```python
from build123d import *

# Parameters (mm, degrees)
SKETCH1_R           = 6.5
SKETCH1_R_2         = 1.5
BOSS_EXTRUDE1_DEPTH = 1.5875
FILLET1_R           = 5


with BuildPart() as part:
    # Sketch1 → Boss-Extrude1 (new body)
    with BuildSketch(Plane.XY):
        Polygon((0, 0), (0, 55), (30, 55), (30, -8.038475773), (-1.519237886, -62.631397208), (-27.5, -47.631397208), align=None)
        with Locations((15, -4.019237886)):
            Circle(SKETCH1_R, mode=Mode.SUBTRACT)
        with Locations((5, 50)):
            Circle(SKETCH1_R_2, mode=Mode.SUBTRACT)
        with Locations((5, 30)):
            Circle(SKETCH1_R_2, mode=Mode.SUBTRACT)
        with Locations((5, 10)):
            Circle(SKETCH1_R_2, mode=Mode.SUBTRACT)
        with Locations(Location((25, 10, 0), (0, 0, 180))):
            Circle(SKETCH1_R_2, mode=Mode.SUBTRACT)
        with Locations(Location((25, 30, 0), (0, 0, 180))):
            Circle(SKETCH1_R_2, mode=Mode.SUBTRACT)
        with Locations(Location((25, 50, 0), (0, 0, 180))):
            Circle(SKETCH1_R_2, mode=Mode.SUBTRACT)
        with Locations((-20.669872981, -45.801270189)):
            Circle(SKETCH1_R_2, mode=Mode.SUBTRACT)
        with Locations((-10.669872981, -28.480762114)):
            Circle(SKETCH1_R_2, mode=Mode.SUBTRACT)
        with Locations((-0.669872981, -11.160254038)):
            Circle(SKETCH1_R_2, mode=Mode.SUBTRACT)
        with Locations(Location((16.650635095, -21.160254038, 0), (0, 0, 180))):
            Circle(SKETCH1_R_2, mode=Mode.SUBTRACT)
        with Locations(Location((6.650635095, -38.480762114, 0), (0, 0, 180))):
            Circle(SKETCH1_R_2, mode=Mode.SUBTRACT)
        with Locations(Location((-3.349364905, -55.801270189, 0), (0, 0, 180))):
            Circle(SKETCH1_R_2, mode=Mode.SUBTRACT)
    extrude(amount=BOSS_EXTRUDE1_DEPTH)

    # Fillet1
    fillet1_edges = [part.edges().sort_by_distance(p)[0] for p in [
        (0, 0, 0.79375),
        (0, 55, 0.79375),
        (30, 55, 0.79375),
        (30, -8.038475773, 0.79375),
        (-1.519237886, -62.631397208, 0.79375),
        (-27.5, -47.631397208, 0.79375),
    ]]
    fillet(fillet1_edges, radius=FILLET1_R)


solid = part.part
```
Could you check a few things on this model? Use its own coordinates, in mm. Give positions to 0.01 mm unless a question says otherwise; leave off trailing zeros. Order: outer loops, then holes, each group sorted by start corner. A loop starts at its lowest first (then second) coordinate and runs counter-clockwise, first axis right, second up.
Q1. If I drill on line 1 along Y through (x, z) = (25, 1); line 2 along X through (y, z) = (29, 1.2); line 3 along Y through (x, z) = (5, 0.55), over which ranges is the centre line in solid material (lowest first)?
Q2. I'm going to push flat-ended pins straight in: P1, Ø2.5, axis at x = 25, y = 50, coming from the -Z side; P2, Ø0.8, axis at y = 33.5, z = 1, coming from the -X side. Where does each tip first touch, or does it pass through?
Q3. Suppose I cut it at B-B, the plane x = 12. Write out the boundary of the cut face in (y, z), and give its area (3 significant figures).
Q4. Suppose I cut it at A-A, the plane y = 30. Write out the boundary of the cut face in (x, z).
Q5. Suppose I cut it at C-C, the plane z = 0.9. Count the separate pieces of the cut face and the enclosed holes in it, and give its area (3 significant figures).
Q6. Suppose I cut it at D-D, the plane x = -17. Write out the boundary of the cut face in (y, z).
Q7. We'd pull the mould along X, two halves only. Please class faces 1 (the flat face through (15.35, -33.41, 0.78)), 2 (the flat face through (3, -2, 0)), 3 (the cylindrical face through (25.325, 51.464, 0.783)): +X half, -X half, draft (parallel to the pull), parting line (faces both ways), or undercut.
Solution:
1. line 1: y = -16.7 to 8.5, 11.5 to 28.5, 31.5 to 48.5, 51.5 to 55
1. line 2: x = 0 to 3.88, 6.12 to 23.88, 26.12 to 30
1. line 3: y = -51.34 to 8.5, 11.5 to 28.5, 31.5 to 48.5, 51.5 to 55
2. P1: passes through
2. P2: stops at x = 0
3. outline: (-39.22, 0) - (-9.79, 0) - (-9.79, 1.59) - (-39.22, 1.59) - close; (1.75, 0) - (55, 0) - (55, 1.59) - (1.75, 1.59) - close
3. area: 131 mm2
4. outline: (0, 0) - (3.5, 0) - (3.5, 1.59) - (0, 1.59) - close; (6.5, 0) - (23.5, 0) - (23.5, 1.59) - (6.5, 1.59) - close; (26.5, 0) - (30, 0) - (30, 1.59) - (26.5, 1.59) - close
5. separate pieces: 1
5. enclosed holes: 13
5. area: 3,300 mm2
6. outline: (-53.69, 0) - (-29.44, 0) - (-29.44, 1.59) - (-53.69, 1.59) - close
7. face 1: +X half
7. face 2: draft
7. face 3: undercut
